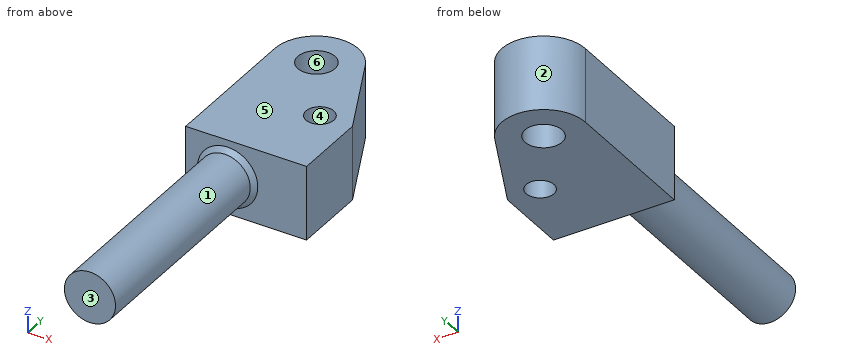
```python
from build123d import *

# Parameters (mm, degrees)
SKETCH1_R           = 5.5
BOSS_EXTRUDE1_DEPTH = 48
SKETCH3_R           = 4
SKETCH3_R_2         = 3
BOSS_EXTRUDE2_DEPTH = 8
CHAMFER1_SIZE       = 1


with BuildPart() as part:
    # Sketch1 → Boss-Extrude1 (new body)
    with BuildSketch(Plane(origin=(0, 0, 0), x_dir=(1, 0, 0), z_dir=(0, 1, 0))):
        with Locations(Location((0, 0, 0), (0, 0, 270))):
            Circle(SKETCH1_R)
    extrude(amount=BOSS_EXTRUDE1_DEPTH)

    # Sketch3 → Boss-Extrude2 (add, symmetric)
    with BuildSketch(Plane.XY):
        with BuildLine():
            Line((0, 48), (17, 48))
            Line((17, 48), (17, 64))
            Line((17, 64), (8.144295771, 82.830201874))
            ThreePointArc((8.144295771, 82.830201874), (-1.962312164, 87.783469188), (-9, 79))
            Line((-9, 79), (-9, 48))
            Line((-9, 48), (0, 48))
        make_face()
        with Locations((0, 79)):
            Circle(SKETCH3_R, mode=Mode.SUBTRACT)
        with Locations((10, 64)):
            Circle(SKETCH3_R_2, mode=Mode.SUBTRACT)
    extrude(amount=BOSS_EXTRUDE2_DEPTH, both=True)

    # Chamfer1
    chamfer1_edges = [part.edges().sort_by_distance(p)[0] for p in [
        (0, 48, -5.5),
    ]]
    chamfer(chamfer1_edges, length=CHAMFER1_SIZE)


solid = part.part
```
Part model, mm, in its own coordinate system. Face numbers are marked on the shaded views. A direction names the side the tool comes from. Coordinates: 2 decimals unless noted, no trailing zeros. Write each loop counter-clockwise with the first axis right and the second up, starting at its lowest first coordinate (ties: lowest second). Pieces come first, ordered by that corner, then holes.
Item 1: Slice it at C-C (y = 5). Write the cut outline in (x, z).
Item 2: Probe line 1 (Y direction, x = 0, z = 3); line 2 (Y direction, x = 10, z = 2.5); line 3 (X direction, y = 61.5, z = 0). List the from-to ranges inside material, lowest first.
Item 3: Which spindle directions (+Z, -Z, +X, -X, +Y, -Y) get a long thin tool onto all of the face, cutting with end or side? Do the marked faces 1 and 2. Say none if no direction does.
Item 4: Slice it at D-D (x = 11). Write the cut outline in (y, z), and give its area (3 significant figures).
Item 5: Slice it at A-A (z = 0). Write the cut outline in (x, y), and give its area (3 significant figures).
Item 6: Pin check, flat tips, straight feed: pin 1 (4 mm diameter, centred on x = -6, y = 25.5, fed in from +Z); pin 2 (5 mm diameter, centred on x = 10, y = 64, fed in from -Z); pin 3 (5 mm diameter, centred on y = 9.5, z = -5, fed in from -X). Stop position of each tip, or through.
Item 7: Mould opens along Y. For the marked faces 3, 4, 5 and 6 say: released by +Y, released by -Y, zero draft, split by the parting line, or undercut.
Item 8: Slice it at B-B (x = 0). Write the cut outline in (y, z).
Results found:
1. outline: circle Ø11 at (0, 0)
2. line 1: y = 0 to 75, 83 to 88
2. line 2: y = 48 to 61, 67 to 78.88
2. line 3: x = -9 to 8.34, 11.66 to 17
3. face 1: -Y
3. face 2: +Z, -Z, +Y
4. outline: (48, -8) - (61.17, -8) - (61.17, 8) - (48, 8) - close; (66.83, -8) - (76.76, -8) - (76.76, 8) - (66.83, 8) - close
4. area: 370 mm2
5. outline: (-9, 48) - (-6.5, 48) - (-5.5, 47) - (-5.5, 0) - (5.5, 0) - (5.5, 47) - (6.5, 48) - (17, 48) - (17, 64) - (8.14, 82.83) arc R9 ccw to (-9, 79) - close; hole circle Ø8 at (0, 79); hole circle Ø6 at (10, 64)
5. area: 1,330 mm2
6. pin 1: stops at z = 3.77
6. pin 2: passes through
6. pin 3: stops at x = -4.9
7. face 3: released by -Y
7. face 4: undercut
7. face 5: zero draft
7. face 6: undercut
8. outline: (0, -5.5) - (47, -5.5) - (48, -6.5) - (48, -8) - (75, -8) - (75, 8) - (48, 8) - (48, 6.5) - (47, 5.5) - (0, 5.5) - close; (83, -8) - (88, -8) - (88, 8) - (83, 8) - close
